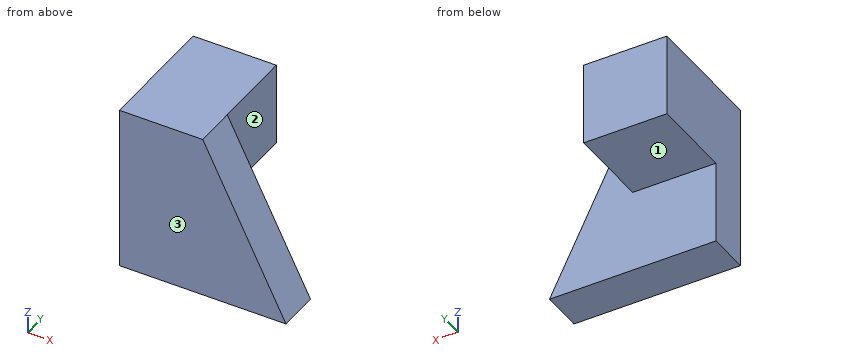
Autodesk Inventor part; units mm, degrees
ref_plane "YZ Plane" through (0, 0, 0) normal (1, 0, 0) x (0, 1, 0)
ref_plane "XZ Plane" through (0, 0, 0) normal (0, 1, 0) x (-1, 0, 0)
ref_plane "XY Plane" through (0, 0, 0) normal (0, 0, 1) x (1, 0, 0)
sketch "草圖1" plane through (0, 0, 0) normal (0, 1, 0) x (-1, 0, 0)
  line L0 (0, 0) -> (20, 0)
  line L1 (20, 0) -> (20, -20)
  line L2 (20, -20) -> (0, -20)
  line L3 (0, -20) -> (0, 0)
  line L4 (20, -20) -> (20, -40)
  line L5 (20, -40) -> (-20, -40)
  line L6 (-20, -40) -> (0, 0)
  dimension "d0" = 20
  dimension "d1" = 20
  dimension "d2" = 20
  dimension "d3" = 40
extrude "擠出1" add sketch "草圖1" along normal blind 30 contours L0 L1 L2 L3
extrude "擠出2" add sketch "草圖1" along normal blind 10 contours L3 L2 L4 L5 L6
Geometry: final body of the model. Coordinates: model frame, mm. Face numbers are marked on the shaded views. A direction names the side the tool comes from. Coordinates: 2 decimals unless noted, no trailing zeros. Loops run counter-clockwise (first coordinate to the right, second up) from the corner with the lowest first, then second, coordinate; pieces in that order, holes last. Notation, with made-up numbers: (55, 11.25) -> (83, 11.25) arc R21 cw to (83, 27.25) -> close; hole circle Ø3 at (-32, 64). An arc over 180 degrees is marked (long way). Use a Markdown table: item, result. Add a question column.
(1) Pin query (flat end, axial travel): pin 1 Ø10 at (y, z) = (17.5, -9) entering from +X; pin 2 Ø6 at (x, z) = (-12, -31.5) entering from +Y; pin 3 Ø1 at (x, y) = (12.5, 7) entering from +Z. Return the tip coordinate at first contact, or that it passes through.
(2) Section query D-D, the plane z = -33.5. Return loops of the section in (x, y), plus the area to 4 significant figures.
(3) Line query: line 1 along X through (y, z) = (12.25, -17.5); line 2 along Y through (x, z) = (-14.5, -26). Output: solid intervals per line, ascending.
(4) Section query B-B, the plane x = -16. Return loops of the section in (y, z), plus the area to 3 significant figures.
(5) Access query for the marked faces 1, 2 and 3. Directions: +Z, -Z, +X, -X, +Y, -Y. A direction counts if a zero-diameter tool reaches every point of the face in a straight line with its end or side. Return the directions, or none.
(6) Section query A-A, the plane z = -3. Return loops of the section in (x, y).
(7) Section query C-C, the plane y = 20. Return loops of the section in (x, z), plus the area to 3 significant figures.
Answer:
| question | item | result |
|---|---|---|
| 1 | pin 1 | stops at x = 0 |
| 1 | pin 2 | stops at y = 10 |
| 1 | pin 3 | stops at z = -24 |
| 2 | outline | (-20, 0) -> (16.75, 0) -> (16.75, 10) -> (-20, 10) -> close |
| 2 | area | 367.5 mm^2 |
| 3 | line 1 | x = -20 to 0 |
| 3 | line 2 | y = 0 to 10 |
| 4 | outline | (0, -40) -> (10, -40) -> (10, -20) -> (30, -20) -> (30, 0) -> (0, 0) -> close |
| 4 | area | 800 mm^2 |
| 5 | face 1 | -Z, +X, -X, +Y |
| 5 | face 2 | +Z, -Z, +X, +Y |
| 5 | face 3 | +Z, -Z, +X, -X, -Y |
| 6 | outline | (-20, 0) -> (1.5, 0) -> (1.5, 10) -> (0, 10) -> (0, 30) -> (-20, 30) -> close |
| 7 | outline | (-20, -20) -> (0, -20) -> (0, 0) -> (-20, 0) -> close |
| 7 | area | 400 mm^2 |
